from build123d import *

# Parameters (mm, degrees)
BOSS_EXTRUDE1_DEPTH = 2.54
BOSS_EXTRUDE2_DEPTH = 1.5875
SKETCH4_R           = 4.7625
CUT_EXTRUDE1_DEPTH  = 134.652038892
SKETCH5_R           = 2.286
CUT_EXTRUDE2_DEPTH  = 134.652038897


with BuildPart() as part:
    # Sketch1 → Boss-Extrude1 (new body)
    with BuildSketch(Plane.XY):
        with BuildLine():
            Line((-1.5875, 91.680354705), (-1.5875, 35.319645295))
            ThreePointArc((-1.5875, 35.319645295), (-2.726536461, 18.348556433), (-6.123214286, 1.681887871))
            ThreePointArc((-6.123214286, 1.681887871), (0, -6.35), (6.123214286, 1.681887871))
            ThreePointArc((6.123214286, 1.681887871), (2.726536461, 18.348556433), (1.5875, 35.319645295))
            Line((1.5875, 35.319645295), (1.5875, 91.680354705))
            ThreePointArc((1.5875, 91.680354705), (2.726536461, 108.651443567), (6.123214286, 125.318112129))
            ThreePointArc((6.123214286, 125.318112129), (0, 133.35), (-6.123214286, 125.318112129))
            ThreePointArc((-6.123214286, 125.318112129), (-2.726536461, 108.651443567), (-1.5875, 91.680354705))
        make_face()
    extrude(amount=BOSS_EXTRUDE1_DEPTH)

    # Sketch3 → Boss-Extrude2 (add, symmetric)
    with BuildSketch(Plane(origin=(0, 0, 0), x_dir=(0, 0, -1), z_dir=(1, 0, 0))):
        with BuildLine():
            Line((-2.54, 0), (-2.54, 127))
            ThreePointArc((-2.54, 127), (-8.89, 63.5), (-2.54, 0))
        make_face()
    extrude(amount=BOSS_EXTRUDE2_DEPTH, both=True)

    # Sketch4 → Cut-Extrude1 (cut, through all)
    with BuildSketch(Plane.XY.offset(2.54)):
        Circle(SKETCH4_R)
        with Locations((0, 127)):
            Circle(SKETCH4_R)
    extrude(amount=CUT_EXTRUDE1_DEPTH, mode=Mode.SUBTRACT)

    # Sketch5 → Cut-Extrude2 (cut, through all)
    with BuildSketch(Plane.XY.offset(2.54)):
        Circle(SKETCH5_R)
        with Locations((0, 127)):
            Circle(SKETCH5_R)
    extrude(amount=-CUT_EXTRUDE2_DEPTH, mode=Mode.SUBTRACT)


solid = part.part
Can you work these out from the model? Positions are in its coordinate system, mm. A direction names the side the tool comes from. Give positions to 0.01 mm unless a question says otherwise; leave off trailing zeros. Order: outer loops, then holes, each group sorted by start corner. A loop starts at its lowest first (then second) coordinate and runs counter-clockwise, first axis right, second up. Notation, with made-up numbers: M 67.5,43.25 L 91.5,43.25 A17 ccw 91.5,61.25 Z; hole C -7.5,31.25 d1. An arc over 180 degrees is marked long. Use one line per item in the form item = value. Start each with the question number.
Item 1: If we section it at A-A (x = 0): State how many separate pieces and enclosed holes the cut face has, then the cut area to 3 significant figures.
Item 2: If I drill on line 1 along Y through (x, z) = (0, 1.25); line 2 along Z through (x, y) = (2.25, 4); line 3 along X through (y, z) = (25, 4.75), over which ranges is the centre line in solid material (lowest first)?
Item 3: We'd pull the mould along Y, two halves only. Please class faces 1 (the flat face through (0, 4, 2.54)), 2 (the cylindrical face through (0.02, 64.33, 8.89)), 3 (the cylindrical face through (-0.5, -2.23, 1.29)): +Y half, -Y half, draft (parallel to the pull), parting line (faces both ways), or undercut.
Item 4: For faces 4 (the cylindrical face through (2.695, 108.415, 1.252)), 5 (the cylindrical face through (-2.76, 108.89, 1.25)), 6 (the flat face through (-1.588, 64, 5)), which set-ups out of +Z, -Z, +X, -X, +Y, -Y let a thin tool reach every point of the face, with its end or its side?
Item 5: If we section it at B-B (y = 0): Write out the boundary of the cut face in (x, z).
Item 6: If we section it at D-D (y = 55): Write out the boundary of the cut face in (x, z), then the cut area to 3 significant figures.
Item 7: Will these pins go through, and if not, where does the flat tip stop? pin 1 Ø4.5 at (y, z) = (52, 3.5) entering from +X; pin 2 Ø6.5 at (x, y) = (-2.5, 12.5) entering from +Z; pin 3 Ø4 at (x, z) = (-4, 4) entering from +Y; pin 4 Ø4 at (x, y) = (0, 127) entering from -Z.
Outcome:
q1.separate_pieces = 3
q1.enclosed_holes = 0
q1.area = 866 mm2
q2.line_1 = -6.35 to -2.29, 2.29 to 124.71, 129.29 to 133.35
q2.line_2 = 0 to 2.54
q2.line_3 = -1.59 to 1.59
q3.face_1 = draft
q3.face_2 = parting line
q3.face_3 = undercut
q4.face_4 = +Z, -Z, +X
q4.face_5 = +Z, -Z, -X
q4.face_6 = +Z, -X
q5.outline = M -6.35,0 L -2.29,0 L -2.29,2.54 L -6.35,2.54 Z; M 2.29,0 L 6.35,0 L 6.35,2.54 L 2.29,2.54 Z
q6.outline = M -1.59,0 L 1.59,0 L 1.59,8.78 L -1.59,8.78 Z
q6.area = 27.9 mm2
q7.pin_1 = 1.59
q7.pin_2 = 5.3
q7.pin_3 = 132.78
q7.pin_4 = through
